from build123d import *

# Parameters (mm, degrees)
SKETCH1_W               = 16
SKETCH1_H               = 16
BOSS_EXTRUDE1_DEPTH     = 12
SKETCH2_W               = 9.5
SKETCH2_H               = 12
BOSS_EXTRUDE2_DEPTH     = 4.5
CIRPATTERN1_COUNT       = 2
CIRPATTERN1_ANGLE       = 90
SKETCH4_W               = 8
SKETCH4_H               = 5.6
BOSS_EXTRUDE3_DEPTH     = 1.5
SKETCH5_W               = 11
SKETCH5_H               = 2.7
BOSS_EXTRUDE4_DEPTH     = 7
SKETCH6_W               = 7
SKETCH6_H               = 6.2
BOSS_EXTRUDE5_DEPTH     = 7
SKETCH7_R               = 6
CUT_EXTRUDE1_DEPTH      = 5
CUT_EXTRUDE2_DEPTH      = 23.918333273
CUT_EXTRUDE2_DEPTH_BACK = 23.918333273
SKETCH8_R               = 0.5
CUT_EXTRUDE3_DEPTH      = 23.918333391
CUT_EXTRUDE3_DEPTH_BACK = 23.918333391
SKETCH9_R               = 0.5
SKETCH10_W              = 1.5
SKETCH10_H              = 0.6
SKETCH10_W_2            = 0.4
SKETCH10_H_2            = 0.8
SKETCH10_W_3            = 0.8
SKETCH10_H_3            = 0.4
SKETCH10_W_4            = 0.7
SKETCH10_H_4            = 0.3
BOSS_EXTRUDE6_DEPTH     = 3.5


with BuildPart() as part:
    # Sketch1 → Boss-Extrude1 (new body)
    with BuildSketch(Plane(origin=(0, 0, 0), x_dir=(1, 0, 0), z_dir=(0, 1, 0))):
        Rectangle(SKETCH1_W, SKETCH1_H)
    extrude(amount=BOSS_EXTRUDE1_DEPTH)

    # Sketch2 → Boss-Extrude2 (add)
    with BuildSketch(Plane.ZY.offset(8)):
        with Locations((0, 6)):
            Rectangle(SKETCH2_W, SKETCH2_H)
    boss_extrude2 = extrude(amount=BOSS_EXTRUDE2_DEPTH)

    # CirPattern1: Boss-Extrude2 ×2 about axis
    cirpattern1_axis = Axis((0, 0, 0), (0, -1, 0))
    for i in range(1, CIRPATTERN1_COUNT):
        add(boss_extrude2.rotate(cirpattern1_axis, i * CIRPATTERN1_ANGLE / (CIRPATTERN1_COUNT - 1)))

    # Sketch4 → Boss-Extrude3 (add)
    with BuildSketch(Plane.XY.offset(8)):
        with Locations((0, 2.8)):
            Rectangle(SKETCH4_W, SKETCH4_H)
    extrude(amount=BOSS_EXTRUDE3_DEPTH)

    # Sketch5 → Boss-Extrude4 (add)
    with BuildSketch(Plane(origin=(8, 0, 0), x_dir=(0, 0, -1), z_dir=(1, 0, 0))):
        with Locations((0, 1.35)):
            Rectangle(SKETCH5_W, SKETCH5_H)
    extrude(amount=BOSS_EXTRUDE4_DEPTH)

    # Sketch6 → Boss-Extrude5 (add)
    with BuildSketch(Plane(origin=(0, 2.7, 0), x_dir=(1, 0, 0), z_dir=(0, 1, 0))):
        with Locations((11.5, 0)):
            Rectangle(SKETCH6_W, SKETCH6_H)
    extrude(amount=BOSS_EXTRUDE5_DEPTH)

    # Sketch7 → Cut-Extrude1 (cut)
    with BuildSketch(Plane(origin=(0, 12, 0), x_dir=(1, 0, 0), z_dir=(0, 1, 0))):
        with Locations(Location((0, 0, 0), (0, 0, 270))):
            Circle(SKETCH7_R)
    extrude(amount=-CUT_EXTRUDE1_DEPTH, mode=Mode.SUBTRACT)

    # Sketch8 → Cut-Extrude2 (cut, two sides: drawn at the far end of the back side and taken through both)
    with BuildSketch(Plane(origin=(0, 0, 0), x_dir=(0, 0, -1), z_dir=(1, 0, 0)).offset(-CUT_EXTRUDE2_DEPTH_BACK)):
        with Locations((0, 7)):
            Circle(SKETCH8_R)
    extrude(amount=CUT_EXTRUDE2_DEPTH + CUT_EXTRUDE2_DEPTH_BACK, mode=Mode.SUBTRACT)

    # Sketch9 → Cut-Extrude3 (cut, two sides: drawn at the far end of the back side and taken through both)
    with BuildSketch(Plane.XY.offset(-CUT_EXTRUDE3_DEPTH_BACK)):
        with Locations(Location((0, 7, 0), (0, 0, 180))):
            Circle(SKETCH9_R)
    extrude(amount=CUT_EXTRUDE3_DEPTH + CUT_EXTRUDE3_DEPTH_BACK, mode=Mode.SUBTRACT)

    # Sketch10 → Boss-Extrude6 (add)
    with BuildSketch(Plane.XZ):
        with Locations((7.25, 7.7)):
            Rectangle(SKETCH10_W, SKETCH10_H)
        with Locations((-7.25, 7.7)):
            Rectangle(SKETCH10_W, SKETCH10_H)
        with Locations((7.25, -7.7)):
            Rectangle(SKETCH10_W, SKETCH10_H)
        with Locations((-7.25, -7.7)):
            Rectangle(SKETCH10_W, SKETCH10_H)
        with Locations((-11.3, 0)):
            Rectangle(SKETCH10_W_2, SKETCH10_H_2)
        with Locations((-11.3, -2.5)):
            Rectangle(SKETCH10_W_2, SKETCH10_H_2)
        with Locations((-11.3, 2.5)):
            Rectangle(SKETCH10_W_2, SKETCH10_H_2)
        with Locations((-2.5, -11.3)):
            Rectangle(SKETCH10_W_3, SKETCH10_H_3)
        with Locations((0, -11.3)):
            Rectangle(SKETCH10_W_3, SKETCH10_H_3)
        with Locations((2.5, -11.3)):
            Rectangle(SKETCH10_W_3, SKETCH10_H_3)
        with Locations((13.15, -3.35)):
            Rectangle(SKETCH10_W_4, SKETCH10_H_4)
        with Locations((8.65, -3.35)):
            Rectangle(SKETCH10_W_4, SKETCH10_H_4)
        with Locations((8.65, 3.05)):
            Rectangle(SKETCH10_W_4, SKETCH10_H_4)
        with Locations((13.15, 3.05)):
            Rectangle(SKETCH10_W_4, SKETCH10_H_4)
    extrude(amount=BOSS_EXTRUDE6_DEPTH)


solid = part.part
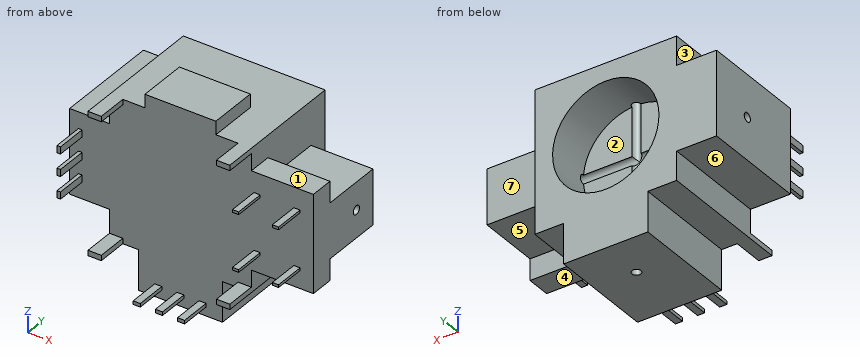
For this review, take the finished solid that the model builds, in its own axes (mm). Face numbers are marked on the shaded views. A direction names the side the tool comes from. Give positions to 0.01 mm unless a question says otherwise; leave off trailing zeros. Order: outer loops, then holes, each group sorted by start corner. A loop starts at its lowest first (then second) coordinate and runs counter-clockwise, first axis right, second up. Notation, with made-up numbers: (9, -15) - (26, -15) arc R18 cw to (26, 17) - close; hole circle Ø5 at (-33, -4). An arc over 180 degrees is marked (long way). Answer as a JSON object with one key per item and string values. Group by question number.
Item 1: Take a section at C-C on y = 3.25. Give the boundary of the cut face in (x, z).
Item 2: Clearance check with flat-ended pins moving along their axes: pin 1 Ø1 at (x, y) = (6, 4) entering from -Z; pin 2 Ø4.5 at (x, z) = (-2.5, -4) entering from +Y; pin 3 Ø0.8 at (x, y) = (8.5, -2) entering from -Z; pin 4 Ø0.6 at (y, z) = (-1, -2.5) entering from +X. State where each tip first meets the part, or that it passes through.
Item 3: Take a section at B-B on x = 9.5. Give the boundary of the cut face in (y, z), and give its area (3 significant figures).
Item 4: Draft analysis for pull direction X (two halves, no side actions). For the marked faces 1, 2 and 3, state which applies: pulls with the +X half, pulls with the -X half, needs draft (parallel to the pull), parting line crosses it, or undercut.
Item 5: Take a section at A-A on y = 11. Give the boundary of the cut face in (x, z).
Item 6: Take a section at D-D on z = 1.75. Give the boundary of the cut face in (x, y), and give its area (3 significant figures).
Item 7: Wall thickness on line 1 along Z through (x, y) = (-10, 7); line 2 along Y through (x, z) = (0, -7.75); line 3 along Z through (x, y) = (0, 10.45): over which ranges is each line inside the solid? List them lowest first.
Item 8: Machinability: for the marked faces 4, 5, 6 and 7, which of the approach directions +Z, -Z, +X, -X, +Y, -Y give a long, thin tool a straight path to every point of the face, cutting with its end or side? Answer none if there is none.
Reported:
{
 "1": {"outline": "(-12.5, -4.75) - (-8, -4.75) - (-8, -8) - (-4.75, -8) - (-4.75, -12.5) - (4.75, -12.5) - (4.75, -8) - (8, -8) - (8, -3.1) - (15, -3.1) - (15, 3.1) - (8, 3.1) - (8, 8) - (4, 8) - (4, 9.5) - (-4, 9.5) - (-4, 8) - (-8, 8) - (-8, 4.75) - (-12.5, 4.75) - close"},
 "2": {"pin 1": "z = -8", "pin 2": "y = 12", "pin 3": "z = -3.5", "pin 4": "x = -11.1"},
 "3": {"outline": "(0, -5.5) - (2.7, -5.5) - (2.7, -3.1) - (9.7, -3.1) - (9.7, 3.1) - (2.7, 3.1) - (2.7, 5.5) - (0, 5.5) - close; hole circle Ø1 at (7, 0)", "area": "72.3 mm^2"},
 "4": {"face 1": "needs draft", "face 2": "undercut", "face 3": "pulls with the -X half"},
 "5": {"outline": "(-12.5, -4.75) - (-8, -4.75) - (-8, -8) - (-4.75, -8) - (-4.75, -12.5) - (4.75, -12.5) - (4.75, -8) - (8, -8) - (8, 8) - (-8, 8) - (-8, 4.75) - (-12.5, 4.75) - close; hole circle Ø12 at (0, 0)"},
 "6": {"outline": "(-12.5, 0) - (15, 0) - (15, 9.7) - (8, 9.7) - (8, 12) - (5.74, 12) - (5.74, 7) - (0.5, 7) arc R0.5 cw to (-0.5, 7) - (-5.74, 7) - (-5.74, 12) - (-12.5, 12) - close", "area": "256 mm^2"},
 "7": {"line 1": "-4.75 to -0.5, 0.5 to 4.75", "line 2": "0 to 6.5, 7.5 to 12", "line 3": "-12.5 to -6, 6 to 8"},
 "8": {"face 4": "-Z, +X, +Y, -Y", "face 5": "-Z, +X, +Y", "face 6": "-Z, -X, +Y, -Y", "face 7": "+Z, -Z, +X, +Y"}
}
